The drawing under review shows one solid part. Ordinate dimensions are in mm from its lowest x, y, z. A direction names the side the tool comes from. Give positions to 0.01 mm unless a question says otherwise; leave off trailing zeros. Write each loop counter-clockwise with the first axis right and the second up, starting at its lowest first coordinate (ties: lowest second). Pieces come first, ordered by that corner, then holes. Notation, with made-up numbers: (19.5, 85.25) -> (67.5, 85.25) arc R24 cw to (67.5, 101.25) -> close; hole circle Ø1 at (-34.5, 56.25). An arc over 180 degrees is marked (long way). Write item = value, one per line.
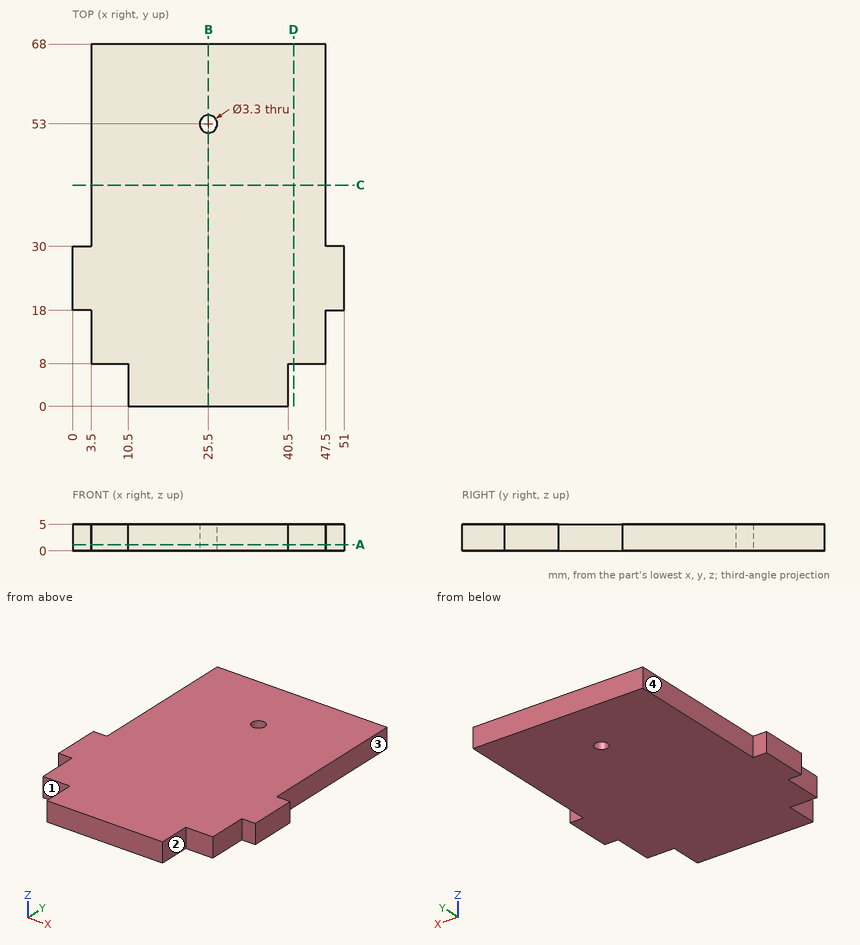
(1) Take a section at B-B (x = 25.5). Write out the cut boundary in (y, z), plus the area to 4 significant figures.
Answers below:
outline = (0, 0) -> (51.35, 0) -> (51.35, 5) -> (0, 5) -> close; (54.65, 0) -> (68, 0) -> (68, 5) -> (54.65, 5) -> close
area = 323.5 mm^2
(2) Take a section at C-C (y = 41.5). Write out the cut boundary in (x, z), plus the area to 3 significant figures.
Answers below:
outline = (3.5, 0) -> (47.5, 0) -> (47.5, 5) -> (3.5, 5) -> close
area = 220 mm^2
(3) To check wall thickness, follow probe 1 along Y at (x, z) = (25.5, 1.7); probe 2 along Y at (x, z) = (5, 2); probe 3 along X at (y, z) = (45.5, 3.15). State the ranges of each line that lie inside material, in increasing order.
Answers below:
probe_1 = 0 to 51.35, 54.65 to 68
probe_2 = 8 to 68
probe_3 = 3.5 to 47.5
(4) Tool access review of the marked faces 1, 2, 3 and 4: name each direction out of +Z, -Z, +X, -X, +Y, -Y from which nothing blocks a thin tool from reaching the whole face with its end or side.
Answers below:
face_1 = +Z, -Z, -X, -Y
face_2 = +Z, -Z, +X, -Y
face_3 = +Z, -Z, +X, +Y
face_4 = +Z, -Z, -X, +Y
(5) Take a section at A-A (z = 1.2). Write out the cut boundary in (x, y).
Answers below:
outline = (0, 18) -> (3.5, 18) -> (3.5, 8) -> (10.5, 8) -> (10.5, 0) -> (40.5, 0) -> (40.5, 8) -> (47.5, 8) -> (47.5, 18) -> (51, 18) -> (51, 30) -> (47.5, 30) -> (47.5, 68) -> (3.5, 68) -> (3.5, 30) -> (0, 30) -> close; hole circle Ø3.3 at (25.5, 53)
(6) Take a section at D-D (x = 41.5). Write out the cut boundary in (y, z), plus the area to 3 significant figures.
Answers below:
outline = (8, 0) -> (68, 0) -> (68, 5) -> (8, 5) -> close
area = 300 mm^2
(7) For pin 1 (1 mm diameter, centred on x = 48.5, z = 1.5, fed in from -Y); pin 2 (2.5 mm diameter, centred on y = 4, z = 3, fed in from -X); pin 3 (1.8 mm diameter, centred on x = 50, z = 2.5, fed in from +Y), all flat-tipped, find the tip position at first contact; note any pin that passes through.
Answers below:
pin_1 = 18
pin_2 = 10.5
pin_3 = 30
